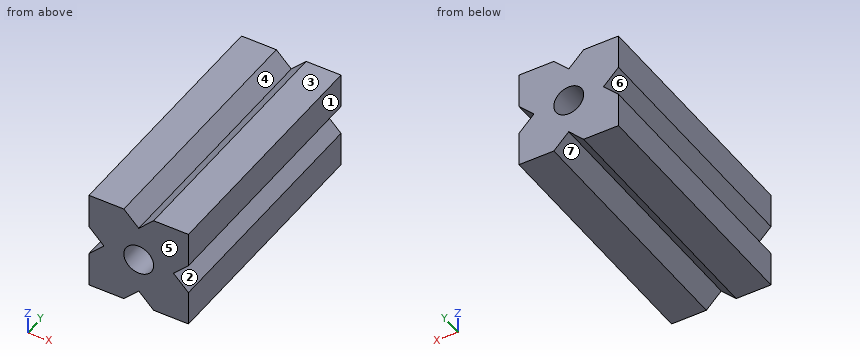
```python
from build123d import *

# Parameters (mm, degrees)
SKIZZE1_W                       = 20
SKIZZE1_H                       = 20
AUFSATZ_LINEAR_AUSTRAGEN1_DEPTH = 25
SCHNITT_LINEAR_AUSTRAGEN1_DEPTH = 51
SKIZZE3_R                       = 3
SCHNITT_LINEAR_AUSTRAGEN2_DEPTH = 51


with BuildPart() as part:
    # Skizze1 → Aufsatz-Linear austragen1 (new body, symmetric)
    with BuildSketch(Plane(origin=(0, 0, 0), x_dir=(1, 0, 0), z_dir=(0, 1, 0))):
        Rectangle(SKIZZE1_W, SKIZZE1_H)
    extrude(amount=AUFSATZ_LINEAR_AUSTRAGEN1_DEPTH, both=True)

    # Skizze2 → Schnitt-Linear austragen1 (cut, through all)
    with BuildSketch(Plane(origin=(0, 25, 0), x_dir=(1, 0, 0), z_dir=(0, 1, 0))):
        Polygon((-3, 10), (0, 7), (3, 10), align=None)
        Polygon((10, 3), (7, 0), (10, -3), align=None)
        Polygon((-10, -3), (-10, 3), (-7, 0), align=None)
        Polygon((-3, -10), (3, -10), (0, -7), align=None)
    extrude(amount=-SCHNITT_LINEAR_AUSTRAGEN1_DEPTH, mode=Mode.SUBTRACT)

    # Skizze3 → Schnitt-Linear austragen2 (cut, through all)
    with BuildSketch(Plane(origin=(0, 25, 0), x_dir=(1, 0, 0), z_dir=(0, 1, 0))):
        Circle(SKIZZE3_R)
    extrude(amount=-SCHNITT_LINEAR_AUSTRAGEN2_DEPTH, mode=Mode.SUBTRACT)


solid = part.part
```
Model file for the job. Use its own axes, mm. Face numbers are marked on the shaded views. A direction names the side the tool comes from. Round coordinates to 2 decimals unless told otherwise and drop trailing zeros. Write each loop counter-clockwise with the first axis right and the second up, starting at its lowest first coordinate (ties: lowest second). Pieces come first, ordered by that corner, then holes. Notation, with made-up numbers: (-1.75, -22) - (26.25, -22) arc R18 cw to (26.25, 3) - close; hole circle Ø6 at (63.5, 0.5). An arc over 180 degrees is marked (long way). Use CSV: the item, a comma, the result in double quotes. Start each with the question number.
Item 1: Band-saw the part on B-B (y = 11). Write the cut outline in (x, z).
Item 2: Tool access for the marked faces 4, 5, 6 and 7: list every direction of +Z, -Z, +X, -X, +Y, -Y with a clear straight run to the whole face (end or side of a thin tool).
Item 3: Pin check, flat tip, straight feed: P1, Ø12, axis at x = 1, y = 15, coming from the -Z side. Stop position of the tip, or through.
Item 4: Band-saw the part on A-A (z = -8.25). Write the cut outline in (x, y), and give its area (3 significant figures).
Item 5: Two-plate mould, pull along Z, no slides. Class the marked faces 1, 2 and 3: released by +Z, released by -Z, zero draft, split by the parting line, or undercut.
Item 6: Drill centre lines: L1, parallel to Z at x = 8.25, y = -8; L2, parallel to X at y = 10, z = -8.5; L3, parallel to Z at x = -8, y = 18. Where is each one in solid material? Low to high. Write a range as [from, to].
Checked values:
1,outline,"(-10, -10) - (-3, -10) - (0, -7) - (3, -10) - (10, -10) - (10, -3) - (7, 0) - (10, 3) - (10, 10) - (3, 10) - (0, 7) - (-3, 10) - (-10, 10) - (-10, 3) - (-7, 0) - (-10, -3) - close; hole circle Ø6 at (0, 0)"
2,face 4,"+Z, +Y, -Y"
2,face 5,"+Z, -Z, +X, -X, -Y"
2,face 6,"-X, +Y, -Y"
2,face 7,"-Z, +Y, -Y"
3,P1,"stops at z = -10"
4,outline,"(-10, -25) - (-1.25, -25) - (-1.25, 25) - (-10, 25) - close; (1.25, -25) - (10, -25) - (10, 25) - (1.25, 25) - close"
4,area,"875 mm²"
5,face 1,"zero draft"
5,face 2,"undercut"
5,face 3,"released by +Z"
6,L1,"z = [-10, -1.25], [1.25, 10]"
6,L2,"x = [-10, -1.5], [1.5, 10]"
6,L3,"z = [-10, -1], [1, 10]"
